from build123d import *

# Parameters (mm, degrees)
BOSS_EXTRUDE1_DEPTH = 3.4
SKETCH1_3_R         = 3.5
BOSS_EXTRUDE2_DEPTH = 6.93
CHAMFER1_SIZE       = 0.5
SKETCH1_4_R         = 3.5
BOSS_EXTRUDE3_DEPTH = 6.93
CHAMFER2_SIZE       = 0.5


with BuildPart() as part:
    # Sketch1 → Boss-Extrude1 (new body)
    with BuildSketch(Plane(origin=(0, 0, 0), x_dir=(1, 0, 0), z_dir=(0, 1, 0))):
        with BuildLine():
            Line((-25.855, 3.98), (25.855, 3.98))
            ThreePointArc((25.855, 3.98), (29.835, 0), (25.855, -3.98))
            Line((25.855, -3.98), (-25.855, -3.98))
            ThreePointArc((-25.855, -3.98), (-29.835, 0), (-25.855, 3.98))
        make_face()
    extrude(amount=BOSS_EXTRUDE1_DEPTH)

    # Sketch1<3> → Boss-Extrude2 (add)
    with BuildSketch(Plane(origin=(0, 0, 0), x_dir=(1, 0, 0), z_dir=(0, 1, 0))):
        with Locations(Location((-16.8275, 0, 0), (0, 0, 90))):
            Circle(SKETCH1_3_R)
        with Locations(Location((16.8275, 0, 0), (0, 0, 90))):
            Circle(SKETCH1_3_R)
    extrude(amount=BOSS_EXTRUDE2_DEPTH)

    # Chamfer1
    chamfer1_edges = [part.edges().sort_by_distance(p)[0] for p in [
        (-16.8275, 6.93, 3.5),
        (16.8275, 6.93, 3.5),
    ]]
    chamfer(chamfer1_edges, length=CHAMFER1_SIZE)

    # Sketch1<4> → Boss-Extrude3 (add)
    with BuildSketch(Plane(origin=(0, 0, 0), x_dir=(1, 0, 0), z_dir=(0, 1, 0))):
        with Locations(Location((0, 0, 0), (0, 0, 90))):
            Circle(SKETCH1_4_R)
    extrude(amount=BOSS_EXTRUDE3_DEPTH)

    # Chamfer2
    chamfer2_edges = [part.edges().sort_by_distance(p)[0] for p in [
        (0, 6.93, 3.5),
    ]]
    chamfer(chamfer2_edges, length=CHAMFER2_SIZE)


solid = part.part
For this review, take the finished solid that the model builds, in its own axes (mm). A direction names the side the tool comes from. Round coordinates to 2 decimals unless told otherwise and drop trailing zeros. Loops run counter-clockwise (first coordinate to the right, second up) from the corner with the lowest first, then second, coordinate; pieces in that order, holes last. Notation, with made-up numbers: (-28, -23) - (18, -23) arc R27 ccw to (18, -1) - close; hole circle Ø10 at (27, 74). An arc over 180 degrees is marked (long way). Put each result on its own line as item: value. Start each with the question number.
1. For probe 1 along X at (y, z) = (5, 0.5); probe 2 along X at (y, z) = (5.75, -1.5); probe 3 along Y at (x, z) = (13, 2.5), list the stretches that pass through material, from the lowest coordinate up. Write a range as [from, to].
2. For faces 1 (the flat face through (0, 2, 3.98)), 2 (the cylindrical face through (13.357, 4.894, 0.456)), list the 3-axis set-ups (+Z, -Z, +X, -X, +Y, -Y) from which the entire face can be reached by the end or side of a thin tool; tool diameter is ignored.
3. Consider section C-C on y = 2. State the section outline as (x, z) points (3 decimals).
4. Insertion check: P1, Ø3, axis at y = 5, z = -2.5, coming from the +X side; P2, Ø2, axis at x = 23, z = 1, coming from the +Y side; P3, Ø4, axis at y = 5.5, z = 2.5, coming from the -X side. Each pin has a flat end and moves straight along its axis. Give the tip position at first contact, or say it passes through.
5. Consider section A-A on z = 0. State the section outline as (x, y) points (1 decimal), plus the area to 3 significant figures.
6. Consider section B-B on x = 0. State the section outline as (y, z) points, plus the area to 3 significant figures.
7. Consider section D-D on x = 23.5. State the section outline as (y, z) points.
Result sheet:
1. probe 1: [-20.29, -13.36], [-3.46, 3.46], [13.36, 20.29]
1. probe 2: [-19.99, -13.67], [-3.16, 3.16], [13.67, 19.99]
1. probe 3: [0, 3.4]
2. face 1: +Z, +X, -X, +Y, -Y
2. face 2: +Y
3. outline: (-25.855, -3.98) - (25.855, -3.98) arc R3.98 ccw to (25.855, 3.98) - (-25.855, 3.98) arc R3.98 ccw to start
4. P1: x = 20.18
4. P2: y = 3.4
4. P3: x = -20.29
5. outline: (-29.8, 0) - (29.8, 0) - (29.8, 3.4) - (20.3, 3.4) - (20.3, 6.4) - (19.8, 6.9) - (13.8, 6.9) - (13.3, 6.4) - (13.3, 3.4) - (3.5, 3.4) - (3.5, 6.4) - (3, 6.9) - (-3, 6.9) - (-3.5, 6.4) - (-3.5, 3.4) - (-13.3, 3.4) - (-13.3, 6.4) - (-13.8, 6.9) - (-19.8, 6.9) - (-20.3, 6.4) - (-20.3, 3.4) - (-29.8, 3.4) - close
5. area: 276 mm^2
6. outline: (0, -3.98) - (3.4, -3.98) - (3.4, -3.5) - (6.43, -3.5) - (6.93, -3) - (6.93, 3) - (6.43, 3.5) - (3.4, 3.5) - (3.4, 3.98) - (0, 3.98) - close
6. area: 51.5 mm^2
7. outline: (0, -3.98) - (3.4, -3.98) - (3.4, 3.98) - (0, 3.98) - close
